Work out the finished part from the listing and answer in its coordinate system (mm). A direction names the side the tool comes from. Give positions to 0.01 mm unless a question says otherwise; leave off trailing zeros. Write each loop counter-clockwise with the first axis right and the second up, starting at its lowest first coordinate (ties: lowest second). Pieces come first, ordered by that corner, then holes. Notation, with made-up numbers: (-14, 15.5) -> (29, 15.5) arc R30 cw to (29, 52.5) -> close; hole circle Ø4 at (20.5, 13). An arc over 180 degrees is marked (long way). Write item = value, one per line. Start each with the question number.
from build123d import *

# Parameters (mm, degrees)
SKETCH2_W           = 40
SKETCH2_H           = 40
BOSS_EXTRUDE1_DEPTH = 3
SKETCH4_W           = 40
SKETCH4_H           = 3
BOSS_EXTRUDE2_DEPTH = 43
FILLET3_R           = 20
CUT_EXTRUDE1_DEPTH  = 37
FILLET4_R           = 1


with BuildPart() as part:
    # Sketch2 → Boss-Extrude1 (new body)
    with BuildSketch(Plane(origin=(0, 0, 0), x_dir=(1, 0, 0), z_dir=(0, 1, 0))):
        Rectangle(SKETCH2_W, SKETCH2_H)
    extrude(amount=BOSS_EXTRUDE1_DEPTH)

    # Sketch4 → Boss-Extrude2 (add)
    with BuildSketch(Plane(origin=(0, 3, 0), x_dir=(1, 0, 0), z_dir=(0, 1, 0))):
        with Locations((0, -18.5)):
            Rectangle(SKETCH4_W, SKETCH4_H)
    extrude(amount=BOSS_EXTRUDE2_DEPTH)

    # Fillet3
    fillet3_edges = [part.edges().sort_by_distance(p)[0] for p in [
        (20, 1.5, -20),
        (-20, 1.5, -20),
    ]]
    fillet(fillet3_edges, radius=FILLET3_R - 0.0001)  # a hair under: the kernel refuses the full size

    # Sketch5 → Cut-Extrude1 (cut)
    with BuildSketch(Plane.XZ):
        with BuildLine():
            Line((6, -7.120873555), (6, 5.305936672))
            ThreePointArc((6, 5.305936672), (1.096488494, 12.934754262), (-5.757118415, 6.995785055))
            Line((-5.757118415, 6.995785055), (-5.757118415, -7.120873555))
            ThreePointArc((-5.757118415, -7.120873555), (0.121440793, -12.999432762), (6, -7.120873555))
        make_face()
    extrude(amount=-CUT_EXTRUDE1_DEPTH, mode=Mode.SUBTRACT)

    # Fillet4
    fillet4_edges = [part.edges().sort_by_distance(p)[0] for p in [
        (20, 3, 8.49995),
        (-20, 24.5, 17),
        (0, 3, 17),
        (20, 24.5, 17),
        (0, 46, 20),
        (0, 46, 17),
        (-20, 3, 8.49995),
        (-14.142164913, 3, -14.142164913),
        (14.142164913, 3, -14.142164913),
        (0, 0, 20),
        (20, 23, 20),
        (-20, 23, 20),
    ]]
    fillet(fillet4_edges, radius=FILLET4_R)


solid = part.part
(1) Each of these flat-tipped pins is pushed along its axis until it touches: pin 1 (6 mm diameter, centred on x = 2.5, y = 27, fed in from -Z); pin 2 (12 mm diameter, centred on x = -0.5, z = 1.5, fed in from +Y); pin 3 (2.5 mm diameter, centred on y = 2, z = -3, fed in from +X). Where does it stop, or does it pass through?
(2) Determine the mould class of faces 4 (the cylindrical face through (14.297, 1.014, -13.986)), 5 (the flat face through (-5.757, 1, 0)), 6 (the flat face through (-20, 11, 18.7)) for opening direction X: pulls with the +X half, pulls with the -X half, needs draft (parallel to the pull), parting line crosses it, or undercut.
(3) A cutting plane is placed at B-B, the plane z = 8.5. Write down the section's boundary in (x, y), then the cut area to 3 significant figures.
(4) For faces 1 (the flat face through (0, 24, 17)), 2 (the flat face through (20, 11, 18.7)), 3 (the cylindrical face through (0, 1, -13)), determine the directions among +Z, -Z, +X, -X, +Y, -Y from which every point of the face is accessible in a straight line to the end or side of a thin tool.
(5) A cutting plane is placed at A-A, the plane y = 20. Write down the section's boundary in (x, z), then the cut area to 3 significant figures.
(6) Find the intervals of material crossed by line 1 along Z through (x, y) = (3, 27); line 2 along Y through (x, z) = (15.5, -3); line 3 along Y through (x, z) = (-11.5, 17.5), in increasing order.
Results list:
q1.pin_1 = 17
q1.pin_2 = 3
q1.pin_3 = 19.92
q2.face_4 = pulls with the +X half
q2.face_5 = undercut
q2.face_6 = pulls with the -X half
q3.outline = (-20, 0) -> (-5.57, 0) -> (-5.57, 3) -> (-19, 3) arc R1 ccw to (-20, 2) -> close; (6.05, 0) -> (20, 0) -> (20, 2) arc R1 ccw to (19, 3) -> (6.05, 3) -> close
q3.area = 84.7 mm²
q4.face_1 = -Z, +X, -X, +Y
q4.face_2 = +Z, -Z, +X, +Y, -Y
q4.face_3 = +Y, -Y
q5.outline = (-20, 18) arc R1 ccw to (-19, 17) -> (19, 17) arc R1 ccw to (20, 18) -> (20, 19) arc R1 ccw to (19, 20) -> (-19, 20) arc R1 ccw to (-20, 19) -> close
q5.area = 119 mm²
q6.line_1 = 17 to 20
q6.line_2 = 0 to 3
q6.line_3 = 0 to 45.87
